```python
from build123d import *

# Parameters (mm, degrees)
SKETCH1_W           = 19
SKETCH1_H           = 19
BOSS_EXTRUDE1_DEPTH = 3.5
CUT_EXTRUDE1_DEPTH  = 4.5
CUT_EXTRUDE2_DEPTH  = 0.6
SKETCH5_W           = 19
SKETCH5_H           = 8
CUT_EXTRUDE3_DEPTH  = 0.6
SKETCH6_R           = 9
CUT_EXTRUDE4_DEPTH  = 1.2
SKETCH7_OUTSIDE_W   = 26.42
SKETCH7_OUTSIDE_H   = 26.42
SKETCH7_OUTSIDE_R   = 1.25
CUT_EXTRUDE5_DEPTH  = 1.3
CUT_EXTRUDE6_DEPTH  = 1
BOSS_EXTRUDE4_DEPTH = 1


with BuildPart() as part:
    # Sketch1 → Boss-Extrude1 (new body)
    with BuildSketch(Plane(origin=(0, 0, 0), x_dir=(1, 0, 0), z_dir=(0, 1, 0))):
        Rectangle(SKETCH1_W, SKETCH1_H)
    extrude(amount=BOSS_EXTRUDE1_DEPTH)

    # Sketch2 → Cut-Extrude1 (cut, through all)
    with BuildSketch(Plane(origin=(0, 3.5, 0), x_dir=(1, 0, 0), z_dir=(0, 1, 0))):
        Polygon((-9.5, -6.812994231), (-6.812994231, -9.5), (-9.5, -9.5), align=None)
    cut_extrude1 = extrude(amount=-CUT_EXTRUDE1_DEPTH, mode=Mode.SUBTRACT)

    # Mirror1: Cut-Extrude1 across plane
    add(cut_extrude1.mirror(Plane(origin=(0, 0, 0), x_dir=(0, 0, 1), z_dir=(1, 0, 0))), mode=Mode.SUBTRACT)

    # Sketch3 → Cut-Extrude2 (cut)
    with BuildSketch(Plane(origin=(0, 3.5, 0), x_dir=(1, 0, 0), z_dir=(0, 1, 0))):
        Polygon((-9.5, 4), (9.5, 4), (9.5, -6.812994231), (6.812994231, -9.5), (-6.812994231, -9.5), (-9.5, -6.812994231), align=None)
    extrude(amount=-CUT_EXTRUDE2_DEPTH, mode=Mode.SUBTRACT)

    # Sketch5 → Cut-Extrude3 (cut)
    with BuildSketch(Plane(origin=(0, 2.9, 0), x_dir=(1, 0, 0), z_dir=(0, 1, 0))):
        Rectangle(SKETCH5_W, SKETCH5_H)
    extrude(amount=-CUT_EXTRUDE3_DEPTH, mode=Mode.SUBTRACT)

    # Sketch6 → Cut-Extrude4 (cut)
    with BuildSketch(Plane(origin=(0, 3.5, 0), x_dir=(1, 0, 0), z_dir=(0, 1, 0))):
        Circle(SKETCH6_R)
    extrude(amount=-CUT_EXTRUDE4_DEPTH, mode=Mode.SUBTRACT)

    # Sketch7 outside → Cut-Extrude5 (cut)
    with BuildSketch(Plane.XZ):
        Rectangle(SKETCH7_OUTSIDE_W, SKETCH7_OUTSIDE_H)
        with Locations((-5.5, -6.20094747)):
            Circle(SKETCH7_OUTSIDE_R, mode=Mode.SUBTRACT)
        with Locations((-5.5, 5.29905253)):
            Circle(SKETCH7_OUTSIDE_R, mode=Mode.SUBTRACT)
        with Locations((5.5, 5.29905253)):
            Circle(SKETCH7_OUTSIDE_R, mode=Mode.SUBTRACT)
        with Locations((5.5, -6.20094747)):
            Circle(SKETCH7_OUTSIDE_R, mode=Mode.SUBTRACT)
    extrude(amount=-CUT_EXTRUDE5_DEPTH, mode=Mode.SUBTRACT)

    # Sketch8 → Cut-Extrude6 (cut)
    with BuildSketch(Plane.XZ.offset(-1.3)):
        with BuildLine():
            Line((-0.6, -9.5), (0.6, -9.5))
            Line((0.6, -9.5), (0.749551834, -5.175923885))
            ThreePointArc((0.749551834, -5.175923885), (0, -4.4), (-0.749551834, -5.175923885))
            Line((-0.749551834, -5.175923885), (-0.6, -9.5))
        make_face()
    cut_extrude6 = extrude(amount=-CUT_EXTRUDE6_DEPTH, mode=Mode.SUBTRACT)

    # Mirror2: Cut-Extrude6 across plane
    add(cut_extrude6.mirror(Plane.XY), mode=Mode.SUBTRACT)

    # Sketch11 → Boss-Extrude4 (add)
    with BuildSketch(Plane.XZ.offset(-1.3)):
        Polygon((-0.6, -9.5), (0.6, -9.5), (0.634585847, -8.5), (-0.634585847, -8.5), align=None)
    boss_extrude4 = extrude(amount=-BOSS_EXTRUDE4_DEPTH)

    # Mirror3: Boss-Extrude4 across plane
    add(boss_extrude4.mirror(Plane.XY))


solid = part.part
```
The listing builds one solid part. Answer for the finished solid, in the listing's coordinates (mm). A direction names the side the tool comes from. Round coordinates to 2 decimals unless told otherwise and drop trailing zeros. Order: outer loops, then holes, each group sorted by start corner. A loop starts at its lowest first (then second) coordinate and runs counter-clockwise, first axis right, second up. Notation, with made-up numbers: (8, 6.25) - (47, 6.25) arc R9 ccw to (47, 11.25) - close; hole circle Ø3 at (89, -21.5). An arc over 180 degrees is marked (long way). Put each result on its own line as item: value. Start each with the question number.
(1) Find section A-A (x = 0). Give the vertices of the cut face in (y, z).
(2) Determine the mould class of faces 6 (the flat face through (8.175, 2.111, 8.138)), 7 (the flat face through (0, 2, -9.5)), 8 (the flat face through (9.5, 2, -1)), 9 (the flat face through (0, 2, -8.5)) for opening direction Z: released by +Z, released by -Z, zero draft, split by the parting line, or undercut.
(3) For faces 1 (the flat face through (-0.1, 3.5, -9.2)), 2 (the flat face through (0, 2, 8.5)), 3 (the flat face through (0, 1.3, 0)), 4 (the flat face through (9, 3, -4)), 5 (the flat face through (0.1, 2.9, 9.2)), determine the directions among +Z, -Z, +X, -X, +Y, -Y from which every point of the face is accessible in a straight line to the end or side of a thin tool.
(4) Given P1, Ø5, axis at x = 3.5, z = -3, coming from the +Y side; P2, Ø4.5, axis at x = 0.5, z = 7, coming from the +Y side; P3, Ø9.5, axis at x = -4, z = -1.5, coming from the -Y side; P4, Ø0.6, axis at x = -9, y = 3, coming from the +Z side, each flat-ended and moving along its own axis, determine where each tip first touches the part or whether it passes through.
(5) Find section C-C (y = 0.7). Give the vertices of the cut face in (x, z).
(6) Find section D-D (x = -5.5). Give the vertices of the cut face in (y, z), plus the area to 3 significant figures.
(7) Straight lines are drawn through the part: probe 1 along Y at (x, z) = (-3, -2.25); probe 2 along Z at (x, y) = (-3.25, 2.8); probe 3 along X at (y, z) = (3.1, -7.5). For each, find the intervals that lie inside material, in ascending order. Write a range as from..to.
(8) Find section B-B (y = 1.9). Give the vertices of the cut face in (x, z), plus the area to 3 significant figures.
Reply:
1. outline: (1.3, -9.5) - (3.5, -9.5) - (3.5, -9) - (2.3, -9) - (2.3, -8.5) - (1.3, -8.5) - close; (1.3, -4.4) - (2.3, -4.4) - (2.3, 4.4) - (1.3, 4.4) - close; (1.3, 8.5) - (2.3, 8.5) - (2.3, 9) - (2.9, 9) - (2.9, 9.5) - (1.3, 9.5) - close
2. face 6: released by +Z
2. face 7: released by -Z
2. face 8: zero draft
2. face 9: undercut
3. face 1: +Z, -Z, +X, -X, +Y
3. face 2: +Y, -Y
3. face 3: -Y
3. face 4: +X, -X, +Y
3. face 5: +Z, +X, -X, +Y
4. P1: y = 2.3
4. P2: y = 2.9
4. P3: y = 0
4. P4: z = 7.6
5. outline: circle Ø2.5 at (-5.5, -6.2); circle Ø2.5 at (-5.5, 5.3); circle Ø2.5 at (5.5, -6.2); circle Ø2.5 at (5.5, 5.3)
6. outline: (0, -7.45) - (1.3, -7.45) - (1.3, -9.5) - (3.5, -9.5) - (3.5, -7.12) - (2.3, -7.12) - (2.3, 7.12) - (2.9, 7.12) - (2.9, 9.5) - (1.3, 9.5) - (1.3, 6.55) - (0, 6.55) - (0, 4.05) - (1.3, 4.05) - (1.3, -4.95) - (0, -4.95) - close
6. area: 29.8 mm^2
7. probe 1: 1.3..2.3
7. probe 2: -9.5..-8.39, 8.39..9.5
7. probe 3: -9.5..-4.97, 4.97..9.5
8. outline: (-9.5, -9.5) - (9.5, -9.5) - (9.5, 6.81) - (6.81, 9.5) - (-6.81, 9.5) - (-9.5, 6.81) - close; hole (-0.75, -5.18) - (-0.63, -8.5) - (0.63, -8.5) - (0.75, -5.18) arc R0.75 ccw (long way) to start; hole (-0.75, 5.18) arc R0.75 ccw (long way) to (0.75, 5.18) - (0.63, 8.5) - (-0.63, 8.5) - close
8. area: 343 mm^2
